For this review, take the finished solid that the model builds, in its own axes (mm). Coordinates: 2 decimals unless noted, no trailing zeros. Loops run counter-clockwise (first coordinate to the right, second up) from the corner with the lowest first, then second, coordinate; pieces in that order, holes last. Notation, with made-up numbers: M -1.5,-5.5 L 35.5,-5.5 A29 cw 35.5,16.5 Z; hole C -24,89 d3. An arc over 180 degrees is marked long. Write each question's results on one line, items separated by ' | '. Start each with the question number.
```python
from build123d import *

# Parameters (mm, degrees)
SKETCH_1_W             = 5
SKETCH_1_H             = 5
EXTRUDE_1_DEPTH        = 5
CUT_EXTRUDE_1_DEPTH    = 5
CHAMFER_1_SIZE2        = 0.070710678
CHAMFER_1_SIZE         = 0.1
CHAMFER_1_EDGE_2_SIZE  = 0.1
CHAMFER_1_EDGE_3_SIZE2 = 0.1
CHAMFER_1_EDGE_3_SIZE  = 0.070710678


with BuildPart() as part:
    # 草图1 → 凸台-拉伸1 (new body)
    with BuildSketch(Plane(origin=(0, 0, 0), x_dir=(1, 0, 0), z_dir=(0, 1, 0))):
        Rectangle(SKETCH_1_W, SKETCH_1_H)
    extrude(amount=EXTRUDE_1_DEPTH)

    # 草图2 → 切除-拉伸1 (cut)
    with BuildSketch(Plane(origin=(0, 5, 0), x_dir=(1, 0, 0), z_dir=(0, 1, 0))):
        Polygon((-2.5, 2.5), (2.5, -2.5), (2.5, 2.5), align=None)
    extrude(amount=-CUT_EXTRUDE_1_DEPTH, mode=Mode.SUBTRACT)

    # 倒角1
    chamfer_1_edges = [part.edges().sort_by_distance(p)[0] for p in [
        (2.5, 2.5, 2.5),
    ]]
    chamfer(chamfer_1_edges, length=CHAMFER_1_SIZE, length2=CHAMFER_1_SIZE2)

    # 倒角1 edge 2
    chamfer_1_edge_2_edges = [part.edges().sort_by_distance(p)[0] for p in [
        (-2.5, 2.5, 2.5),
    ]]
    chamfer(chamfer_1_edge_2_edges, length=CHAMFER_1_EDGE_2_SIZE)

    # 倒角1 edge 3
    chamfer_1_edge_3_edges = [part.edges().sort_by_distance(p)[0] for p in [
        (-2.5, 2.5, -2.5),
    ]]
    chamfer(chamfer_1_edge_3_edges, length=CHAMFER_1_EDGE_3_SIZE, length2=CHAMFER_1_EDGE_3_SIZE2)


solid = part.part
```
Q1. Take a section at C-C, the plane y = 4.7. Give the boundary of the cut face in (x, z), then the cut area to 3 significant figures.
Q2. Take a section at A-A, the plane z = -0.6. Give the boundary of the cut face in (x, y).
Q3. To check wall thickness, follow line 1 along X through (y, z) = (0.55, 0); line 2 along Z through (x, y) = (-0.05, 0.35); line 3 along X through (y, z) = (4.2, 0.1). State the ranges of each line that lie inside material, in increasing order.
Q4. Insertion check: P1, Ø2, axis at y = 2, z = 1, coming from the +X side; P2, Ø2, axis at x = 1, y = 2, coming from the -Z side. Each pin has a flat end and moves straight along its axis. Give the tip position at first contact, or say it passes through.
Q5. Take a section at B-B, the plane x = -1.6. Give the boundary of the cut face in (y, z), then the cut area to 3 significant figures.
Results:
1) outline: M -2.5,-2.43 L -2.43,-2.43 L 2.45,2.45 L 2.4,2.5 L -2.4,2.5 L -2.5,2.4 Z | area: 12.5 mm^2
2) outline: M -2.5,0 L -0.6,0 L -0.6,5 L -2.5,5 Z
3) line 1: -2.5 to 0 | line 2: -0.05 to 2.5 | line 3: -2.5 to 0.1
4) P1: x = 2 | P2: z = 0
5) outline: M 0,-1.6 L 5,-1.6 L 5,2.5 L 0,2.5 Z | area: 20.5 mm^2
